```python
from build123d import *

# Parameters (mm, degrees)
FILLET1_R = 0.5


with BuildPart() as part:
    # Sketch1 → Revolve1 (revolve)
    with BuildSketch(Plane.XY):
        with BuildLine():
            Line((-14.176, 22), (-25, 0))
            ThreePointArc((-25, 0), (-21.46926352, -12.809009482), (-11.874342087, -22))
            Line((-11.874342087, -22), (-5, -22))
            Line((-5, -22), (-5, 0))
            Line((-5, 0), (-2.5, 0))
            Line((-2.5, 0), (-2.5, 20))
            Line((-2.5, 20), (-12.7, 20))
            Line((-12.7, 20), (-12.7, 22))
            Line((-12.7, 22), (-14.176, 22))
        make_face()
    revolve(axis=Axis((0, 0, 0), (0, -1, 0)))

    # Fillet1
    fillet1_edges = [part.edges().sort_by_distance(p)[0] for p in [
        (5, -22, 0),
        (11.874342087, -22, 0),
    ]]
    fillet(fillet1_edges, radius=FILLET1_R)


solid = part.part
```
Read the model definition and answer for the solid it produces. Units are mm, in the model's axes. A direction names the side the tool comes from. Give positions to 0.01 mm unless a question says otherwise; leave off trailing zeros. Order: outer loops, then holes, each group sorted by start corner. A loop starts at its lowest first (then second) coordinate and runs counter-clockwise, first axis right, second up.
(1) Find section B-B (y = 2). Give the vertices of the cut face in (x, z).
(2) For faces 4 (the flat face through (-2, 0, 2)), 5 (the flat face through (3, 20, 0)), 6 (the flat face through (-13, 22, 1)), determine the directions among +Z, -Z, +X, -X, +Y, -Y from which every point of the face is accessible in a straight line to the end or side of a thin tool.
(3) Given pin 1 (1 mm diameter, centred on x = 3, y = -1.5, fed in from -Z); pin 2 (15 mm diameter, centred on x = 0, z = 0, fed in from +Y); pin 3 (3 mm diameter, centred on y = -12.5, z = -19.5, fed in from +X), each flat-ended and moving along its own axis, determine where each tip first touches the part or whether it passes through.
(4) For a pull along X with two mould halves and no side action, classify faces 1 (the conical face through (3.481, 18.179, 15.674)), 2 (the cylindrical face through (0.54, 10.14, 2.44)), 3 (the flat face through (-5, -22, 3)) as released by +X, released by -X, zero draft, split by the parting line, or undercut.
(5) Straight lines are drawn through the part: L1, parallel to X at y = -14, z = 0; L2, parallel to X at y = 21.25, z = 0 (3 decimals); L3, parallel to Z at x = 1.5, y = 5. For each, find the intervals that lie inside material, in ascending order.
(6) Find section A-A (y = -16). Give the vertices of the cut face in (x, z).
Result sheet:
1. outline: circle Ø48.03 at (0, 0); hole circle Ø5 at (0, 0)
2. face 4: -Y
2. face 5: +Y
2. face 6: +Z, -Z, +X, -X, +Y
3. pin 1: stops at z = -24.84
3. pin 2: stops at y = 20
3. pin 3: stops at x = 12.48
4. face 1: split by the parting line
4. face 2: undercut
4. face 3: zero draft
5. L1: x = -20.71 to -5, 5 to 20.71
5. L2: x = -14.545 to -12.7, 12.7 to 14.545
5. L3: z = -22.49 to -2, 2 to 22.49
6. outline: circle Ø38.42 at (0, 0); hole circle Ø10 at (0, 0)
